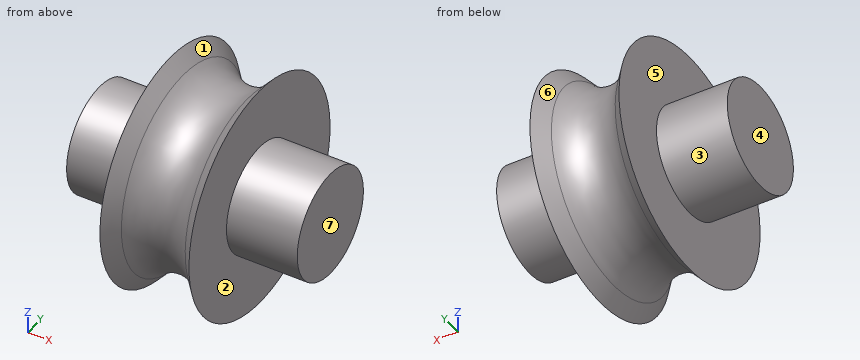
from build123d import *


with BuildPart() as f1:
    # F0 (on Front) → F1 (revolve)
    with BuildSketch(Plane.XZ):
        with BuildLine():
            Line((25.6159, 0), (25.6159, 11.90625))
            Line((25.6159, 11.90625), (9.887509, 11.90625))
            Line((9.887509, 11.90625), (9.887509, 25.4))
            Line((9.887509, 25.4), (7.086038, 22.225))
            ThreePointArc((7.086038, 22.225), (0, 19.027293), (-7.086038, 22.225))
            Line((-7.086038, 22.225), (-9.887509, 25.4))
            Line((-9.887509, 25.4), (-9.887509, 11.90625))
            Line((-9.887509, 11.90625), (-25.6159, 11.90625))
            Line((-25.6159, 11.90625), (-25.6159, 0))
            Line((-25.6159, 0), (25.6159, 0))
        make_face()
    revolve(axis=Axis((0, 0, 0), (1, 0, 0)))


solid = f1.part
The model under review builds one solid part; all positions refer to its coordinate system, in mm. Face numbers are marked on the shaded views. A direction names the side the tool comes from. Give positions to 0.01 mm unless a question says otherwise; leave off trailing zeros. Loops run counter-clockwise (first coordinate to the right, second up) from the corner with the lowest first, then second, coordinate; pieces in that order, holes last. Notation, with made-up numbers: (-9, 58.25) -> (37, 58.25) arc R22 cw to (37, 77.25) -> close; hole circle Ø1 at (42.25, 30.5). An arc over 180 degrees is marked (long way). Answer as a JSON object with one key per item and string values. Group by question number.
Q1. Wall thickness on line 1 along X through (y, z) = (15, 7); line 2 along X through (y, z) = (4, -21.5); line 3 along X through (y, z) = (-20, 0.5): over which ranges is each line inside the solid? List them lowest first.
Q2. Draft analysis for pull direction X (two halves, no side actions). For the marked faces 5, 6 and 7, state which applies: pulls with the +X half, pulls with the -X half, needs draft (parallel to the pull), parting line crosses it, or undercut.
Q3. Take a section at D-D (x = -8.5). Write out the cut boundary in (y, z).
Q4. Tool access review of the marked faces 1, 2, 3 and 4: name each direction out of +Z, -Z, +X, -X, +Y, -Y from which nothing blocks a thin tool from reaching the whole face with its end or side.
Q5. Insertion check: pin 1 (4 mm diameter, centred on x = 16, z = 8, fed in from +Y); pin 2 (10 mm diameter, centred on x = 2.5, z = 4, fed in from +Y); pin 3 (10 mm diameter, centred on x = -3.5, z = 18.5, fed in from -Y). Each pin has a flat end and moves straight along its axis. Give the tip position at first contact, or say it passes through.
Q6. Take a section at C-C (x = -18). Write out the cut boundary in (y, z), plus the area to 3 significant figures.
Q7. Take a section at A-A (z = 0). Write out the cut boundary in (x, y) (1 decimal), plus the area to 3 significant figures.
Answer below:
{
 "1": {"line 1": "x = -9.89 to 9.89", "line 2": "x = -9.89 to -6.76, 6.76 to 9.89", "line 3": "x = -9.89 to -4.19, 4.19 to 9.89"},
 "2": {"face 5": "pulls with the -X half", "face 6": "undercut", "face 7": "pulls with the +X half"},
 "3": {"outline": "circle Ø47.65 at (0, 0)"},
 "4": {"face 1": "none", "face 2": "+X", "face 3": "-X", "face 4": "+Z, -Z, -X, +Y, -Y"},
 "5": {"pin 1": "stops at y = 10.28", "pin 2": "stops at y = 22.4", "pin 3": "stops at y = -16.62"},
 "6": {"outline": "circle Ø23.81 at (0, 0)", "area": "445 mm2"},
 "7": {"outline": "(-25.6, -11.9) -> (-9.9, -11.9) -> (-9.9, -25.4) -> (-7.1, -22.2) arc R9.5 cw to (7.1, -22.2) -> (9.9, -25.4) -> (9.9, -11.9) -> (25.6, -11.9) -> (25.6, 11.9) -> (9.9, 11.9) -> (9.9, 25.4) -> (7.1, 22.2) arc R9.5 cw to (-7.1, 22.2) -> (-9.9, 25.4) -> (-9.9, 11.9) -> (-25.6, 11.9) -> close", "area": "1,580 mm2"}
}
